from build123d import *

# Parameters (mm, degrees)
BOSS_EXTRUDE1_DEPTH = 3


with BuildPart() as part:
    # Model → Boss-Extrude1 (new body)
    with BuildSketch(Plane.XY):
        with BuildLine():
            Line((37.008, 72.936), (25.508, 72.936))
            Line((25.508, 72.936), (25.508, 64.936))
            Line((25.508, 64.936), (28.508, 64.936))
            Line((28.508, 64.936), (28.508, 52.436))
            Line((28.508, 52.436), (32.508, 52.436))
            Line((32.508, 52.436), (32.508, 53.736))
            Line((32.508, 53.736), (35.508, 53.736))
            Line((35.508, 53.736), (35.508, 52.436))
            Line((35.508, 52.436), (37.508, 52.436))
            Line((37.508, 52.436), (37.508, 49.436))
            Line((37.508, 49.436), (35.508, 49.436))
            Line((35.508, 49.436), (35.508, 48.136))
            Line((35.508, 48.136), (32.508, 48.136))
            Line((32.508, 48.136), (32.508, 49.436))
            Line((32.508, 49.436), (28.508, 49.436))
            Line((28.508, 49.436), (28.508, 34.936))
            Line((28.508, 34.936), (25.508, 34.936))
            Line((25.508, 34.936), (25.508, 30.436))
            Line((25.508, 30.436), (25.508, 25.936))
            Line((25.508, 25.936), (28.7315, 25.936))
            ThreePointArc((28.7315, 25.936), (30.43997083, 25.380193402), (31.569029282, 23.982688281))
            ThreePointArc((31.569029282, 23.982688281), (32.427770148, 21.524625278), (32.708, 18.936))
            Line((32.708, 18.936), (32.708, 12.936))
            Line((32.708, 12.936), (49.308, 12.936))
            Line((49.308, 12.936), (49.308, 20.436))
            Line((49.308, 20.436), (46.308, 20.436))
            Line((46.308, 20.436), (46.308, 33.436))
            Line((46.308, 33.436), (42.308, 33.436))
            Line((42.308, 33.436), (42.308, 32.136))
            Line((42.308, 32.136), (39.308, 32.136))
            Line((39.308, 32.136), (39.308, 33.436))
            Line((39.308, 33.436), (37.308, 33.436))
            Line((37.308, 33.436), (37.308, 36.436))
            Line((37.308, 36.436), (39.308, 36.436))
            Line((39.308, 36.436), (39.308, 37.736))
            Line((39.308, 37.736), (42.308, 37.736))
            Line((42.308, 37.736), (42.308, 36.436))
            Line((42.308, 36.436), (46.308, 36.436))
            Line((46.308, 36.436), (46.308, 67.936))
            Line((46.308, 67.936), (49.308, 67.936))
            Line((49.308, 67.936), (49.308, 72.936))
            Line((49.308, 72.936), (37.008, 72.936))
        make_face()
        with BuildLine():
            Line((41.008, 57.1861), (34.008, 57.1861))
            ThreePointArc((34.008, 57.1861), (32.593735358, 57.771764643), (32.008, 59.186))
            Line((32.008, 59.186), (32.008, 67.436))
            ThreePointArc((32.008, 67.436), (32.7402, 69.2038), (34.508, 69.936))
            Line((34.508, 69.936), (40.508, 69.936))
            ThreePointArc((40.508, 69.936), (42.27578125, 69.20378125), (43.008, 67.436))
            Line((43.008, 67.436), (43.008, 59.186))
            ThreePointArc((43.008, 59.186), (42.422214645, 57.771814644), (41.008, 57.1861))
        make_face(mode=Mode.SUBTRACT)
    extrude(amount=BOSS_EXTRUDE1_DEPTH)


solid = part.part
Work out the finished part from the listing and answer in its coordinate system (mm). A direction names the side the tool comes from. Coordinates: 2 decimals unless noted, no trailing zeros. Loops run counter-clockwise (first coordinate to the right, second up) from the corner with the lowest first, then second, coordinate; pieces in that order, holes last. Notation, with made-up numbers: M -32,19.25 L 23,19.25 A33 cw 23,56.25 Z; hole C -4.75,85 d8. An arc over 180 degrees is marked long. Answer in a Markdown table with one row per item. Add a question column.
1. Find section B-B, the plane x = 47.25. Write down the section's boundary in (y, z), then the cut area to 3 significant figures.
2. Find section C-C, the plane x = 38.5. Write down the section's boundary in (y, z), then the cut area to 3 significant figures.
3. Consider L1, parallel to Y at x = 36, z = 2.4; L2, parallel to Y at x = 40.75, z = 0.35; L3, parallel to Y at x = 27, z = 2.2. Determine where each line is inside the solid, lowest interval first.
4. Find section A-A, the plane y = 65.5. Write down the section's boundary in (x, z), then the cut area to 3 significant figures.
5. The mould has two halves that part along X. Classify faces 1 (the flat face through (38, 33.436, 1)), 2 (the flat face through (35.508, 53, 1)), 3 (the flat face through (39.308, 33, 1)), 4 (the flat face through (37.508, 51, 1)): pulls with the +X half, pulls with the -X half, needs draft (parallel to the pull), parting line crosses it, or undercut.
6. Flat-ended cylindrical pins translate along their axes: P1, Ø1, axis at y = 30, z = 0.5, coming from the +X side; P2, Ø0.9, axis at y = 51, z = 1.5, coming from the -X side; P3, Ø1.5, axis at y = 15, z = 1.5, coming from the -X side. Find the tip coordinate at first contact, or state that the pin passes through.
7. Find section D-D, the plane y = 44.5. Write down the section's boundary in (x, z).
8. A tool of negligible diameter and unlimited length cuts with its end or side. For faces 5 (the flat face through (28.508, 42, 1)), 6 (the flat face through (44, 33.436, 1)), 7 (the flat face through (32.708, 16, 1)), 8 (the cylindrical face through (42.44, 57.79, 1.48)), from which of +Z, -Z, +X, -X, +Y, -Y can it reach the whole face along a straight path? Write none if from no direction.
Reported:
| question | item | result |
|---|---|---|
| 1 | outline | M 12.94,0 L 20.44,0 L 20.44,3 L 12.94,3 Z; M 67.94,0 L 72.94,0 L 72.94,3 L 67.94,3 Z |
| 1 | area | 37.5 mm^2 |
| 2 | outline | M 12.94,0 L 33.44,0 L 33.44,3 L 12.94,3 Z; M 36.44,0 L 57.19,0 L 57.19,3 L 36.44,3 Z; M 69.94,0 L 72.94,0 L 72.94,3 L 69.94,3 Z |
| 2 | area | 133 mm^2 |
| 3 | L1 | y = 12.94 to 49.44, 52.44 to 57.19, 69.94 to 72.94 |
| 3 | L2 | y = 12.94 to 32.14, 37.74 to 57.19, 69.92 to 72.94 |
| 3 | L3 | y = 25.94 to 34.94, 64.94 to 72.94 |
| 4 | outline | M 25.51,0 L 32.01,0 L 32.01,3 L 25.51,3 Z; M 43.01,0 L 46.31,0 L 46.31,3 L 43.01,3 Z |
| 4 | area | 29.4 mm^2 |
| 5 | face 1 | needs draft |
| 5 | face 2 | undercut |
| 5 | face 3 | undercut |
| 5 | face 4 | pulls with the -X half |
| 6 | P1 | stops at x = 46.31 |
| 6 | P2 | stops at x = 37.51 |
| 6 | P3 | stops at x = 32.71 |
| 7 | outline | M 28.51,0 L 46.31,0 L 46.31,3 L 28.51,3 Z |
| 8 | face 5 | +Z, -Z, -X |
| 8 | face 6 | +Z, -Z, +X |
| 8 | face 7 | +Z, -Z, -X, -Y |
| 8 | face 8 | +Z, -Z |
